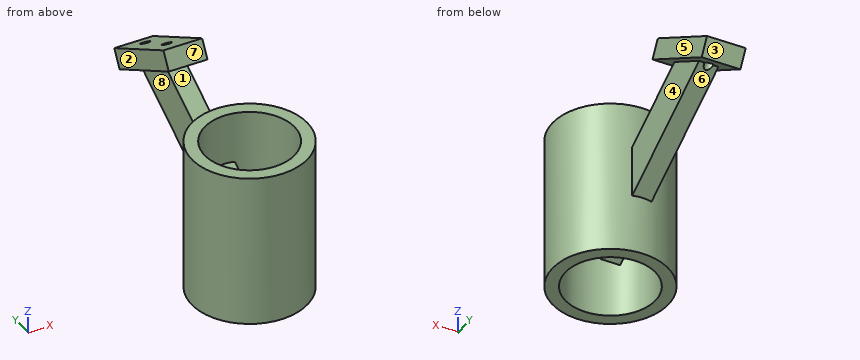
```python
from build123d import *

# Parameters (mm, degrees)
F0_R     = 28.575
F0_R_2   = 22.225
F1_DEPTH = 76.2
F3_DEPTH = 4.7625
F4_W     = 19.05
F4_H     = 50.8
F5_DEPTH = 9.525
F6_R     = 2.286
F7_DEPTH = 25.4


with BuildPart() as f1:
    # F0 (on Top) → F1 (new body)
    with BuildSketch(Plane.XY):
        Circle(F0_R)
        Circle(F0_R_2, mode=Mode.SUBTRACT)
    extrude(amount=F1_DEPTH)

    # F2 (on Right) → F3 (join, symmetric)
    with BuildSketch(Plane.YZ):
        Polygon((0, 38.120868), (0, 12.720868), (87.988181, 63.520868), (65.991136, 76.220868), align=None)
    extrude(amount=F3_DEPTH, both=True)

    # F4 (on face) → F5 (join)
    with BuildSketch(Plane(origin=(0, 49.502388, 85.740651), x_dir=(1, 0, 0), z_dir=(0, 0.5, 0.866025))):
        with Locations((0, 31.739566)):
            Rectangle(F4_W, F4_H)
    extrude(amount=F5_DEPTH)

    # F6 (on face) → F7 (cut)
    with BuildSketch(Plane(origin=(0, 54.264888, 93.989543), x_dir=(1, 0, 0), z_dir=(0, 0.5, 0.866025))):
        with Locations((0, 22.913066)):
            Circle(F6_R)
        with Locations((0, 45.138066)):
            Circle(F6_R)
    extrude(amount=-F7_DEPTH, mode=Mode.SUBTRACT)


solid = f1.part
```
Verification items for the finished model (mm, model axes). Face numbers are marked on the shaded views. A direction names the side the tool comes from. Round coordinates to 2 decimals unless told otherwise and drop trailing zeros. Loops run counter-clockwise (first coordinate to the right, second up) from the corner with the lowest first, then second, coordinate; pieces in that order, holes last. Notation, with made-up numbers: (-29.75, 58) -> (-17.75, 58) arc R10 ccw to (-17.75, 68) -> close; hole circle Ø9 at (49.5, 12). An arc over 180 degrees is marked (long way). Answer as a JSON object with one key per item and string values.
Q1. Scan lines: line 1 (Y direction, x = 0, z = 24) (3 decimals); line 2 (Y direction, x = 0, z = 33.5) (3 decimals); line 3 (X direction, y = 66, z = 75.5). Record each from-to range of solid material in increasing order. Write a range as from..to.
Data:
{"line 1": "y = -28.575..-22.225, 0..19.536, 22.225..28.575", "line 2": "y = -28.575..-22.225, 0..35.991", "line 3": "x = -4.76..4.76"}
Q2. Section check D-D (y = 16.5). Record the boundary of the cut face in (x, z), then the cut area to 3 significant figures.
Data:
{"outline": "(-23.33, 0) -> (-14.89, 0) -> (-14.89, 76.2) -> (-23.33, 76.2) -> close; (-4.76, 22.25) -> (4.76, 22.25) -> (4.76, 47.65) -> (-4.76, 47.65) -> close; (14.89, 0) -> (23.33, 0) -> (23.33, 76.2) -> (14.89, 76.2) -> close", "area": "1,530 mm2"}
Q3. Section check C-C (x = 16.5). Record the boundary of the cut face in (y, z), then the cut area to 3 significant figures.
Data:
{"outline": "(-23.33, 0) -> (-14.89, 0) -> (-14.89, 76.2) -> (-23.33, 76.2) -> close; (14.89, 0) -> (23.33, 0) -> (23.33, 76.2) -> (14.89, 76.2) -> close", "area": "1,290 mm2"}
Q4. Access from +Z, -Z, +X, -X, +Y, -Y to the whole of each face (thin tool, end or side, straight path). Record for the marked faces 4, 5, 6, 7 and 8.
Data:
{"face 4": "-Z, +X", "face 5": "+Z, -Z, +X, +Y", "face 6": "-Z, +X, -X", "face 7": "+Z, +X, -X, -Y", "face 8": "-Z, -X"}
Q5. Go/stop test with flat-tipped pins: P1, Ø4, axis at y = 3.5, z = 9.5, coming from the -X side; P2, Ø10, axis at y = 7.5, z = 30.5, coming from the +X side; P3, Ø2, axis at x = -2.5, y = 53.5, coming from the -Z side. Record where each tip stops, or that it passes through.
Data:
{"P1": "stops at x = -28.54", "P2": "stops at x = 28.47", "P3": "stops at z = 43.03"}
Q6. Section check B-B (x = 0). Record the boundary of the cut face in (y, z) (1 decimal), then the cut area to 3 significant figures.
Data:
{"outline": "(-28.6, 0) -> (-22.2, 0) -> (-22.2, 76.2) -> (-28.6, 76.2) -> close; (0, 12.7) -> (22.2, 25.6) -> (22.2, 0) -> (28.6, 0) -> (28.6, 29.2) -> (85.2, 61.9) -> (91.4, 72.6) -> (76.1, 81.4) -> (63.4, 59.4) -> (59.4, 61.7) -> (72.1, 83.7) -> (59.8, 90.8) -> (55, 82.6) -> (66, 76.2) -> (28.6, 54.6) -> (28.6, 76.2) -> (22.2, 76.2) -> (22.2, 51) -> (0, 38.1) -> close; (90.6, 62) -> (99, 57.2) -> (103.7, 65.4) -> (95.3, 70.3) -> close", "area": "3,080 mm2"}
Q7. Draft check along Z on the marked faces 1, 2 and 3. Enter one of: pulls with the +Z half, pulls with the -Z half, needs draft (parallel to the pull), parting line crosses it, or undercut.
Data:
{"face 1": "undercut", "face 2": "needs draft", "face 3": "pulls with the -Z half"}
